```python
from build123d import *

# Parameters (mm, degrees)
F2_W     = 15
F2_H     = 15
F3_DEPTH = 3
F4_R     = 3


with BuildPart() as f1:
    # F0 (on Top) → F1 (revolve)
    with BuildSketch(Plane.XY):
        with BuildLine():
            Line((-12, 0), (0, 0))
            Line((0, 0), (0, 12))
            ThreePointArc((0, 12), (-8.485281, 8.485281), (-12, 0))
        make_face()
    revolve(axis=Axis((0, 6, 0), (0, 1, 0)))

    # F2 (on Front) → F3 (join)
    with BuildSketch(Plane.XZ):
        with Locations((-7.5, -7.5)):
            Rectangle(F2_W, F2_H)
        Polygon((14.947975, 0), (0, 0), (0, -15), (15, -15), (15, 0), align=None)
        Polygon((-15, 0), (0, 0), (14.947975, 0), (15, 0), (15, 15), (-15, 15), align=None)
    extrude(amount=F3_DEPTH)

    # F4
    f4_edges = [f1.edges().sort_by_distance(p)[0] for p in [
        (15, -1.5, 15),
        (15, -1.5, -15),
        (-15, -1.5, -15),
        (-15, -1.5, 15),
        (12, 0, 0),
    ]]
    fillet(f4_edges, radius=F4_R)


solid = f1.part
```
The model under review builds one solid part; all positions refer to its coordinate system, in mm. A direction names the side the tool comes from. Round coordinates to 2 decimals unless told otherwise and drop trailing zeros. One line per item, written item: value. Start each with the question number.
Q1. Wall thickness on line 1 (Y direction, x = 9.5, z = -12); line 2 (X direction, y = 1.25, z = -9); line 3 (X direction, y = 6, z = 1): over which ranges is each line inside the solid? List them lowest first.
Q2. Machinability: for faces 1 (the face through (-14.14, -1.52, 14.1)), 2 (the face through (-6, 0, -14)), which of the approach directions +Z, -Z, +X, -X, +Y, -Y give a long, thin tool a straight path to every point of the face, cutting with its end or side? Answer none if there is none.
Q3. Clearance check with flat-ended pins moving along their axes: pin 1 Ø2 at (x, y) = (-2, 2.5) entering from +Z; pin 2 Ø3 at (x, y) = (-5.5, 9.5) entering from +Z; pin 3 Ø3 at (y, z) = (3.5, -8) entering from +X. State where each tip first meets the part, or that it passes through.
Reported:
1. line 1: y = -3 to 0
1. line 2: x = -8.33 to 8.33
1. line 3: x = -10.34 to 10.34
2. face 1: +Z, -X, +Y, -Y
2. face 2: +Y
3. pin 1: stops at z = 11.95
3. pin 2: stops at z = 7.36
3. pin 3: stops at x = 9.58
